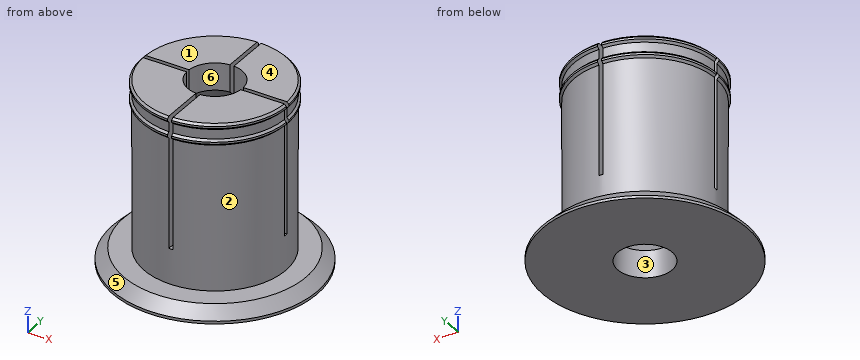
```python
from build123d import *

# Parameters (mm, degrees)
AXLE_BASE_SKETCH_R        = 26
AXLE_DEPTH                = 61.5
GUARD_BASE_R              = 37.5
GUARD_DEPTH               = 5
INNER_AXLE_HOLE_BASE_R    = 10
INNER_AXLE_HOLE_DEPTH     = 67.5
BEND_START                = -48.5
BEND_ROOM_BASE_W          = 1.5
BEND_ROOM_BASE_H          = 75
BEND_ROOM_1_DEPTH         = 48.5
BEND_ROOM_2_COUNT         = 2
BEND_ROOM_2_ANGLE         = 90
EASY_REMOVAL_CHAMFER_SIZE = 4


with BuildPart() as part:
    # Axle base sketch → Axle (new body)
    with BuildSketch(Plane.XY):
        Circle(AXLE_BASE_SKETCH_R)
    extrude(amount=AXLE_DEPTH)

    # Guard base → Guard (add)
    with BuildSketch(Plane(origin=(0, 0, 0), x_dir=(-1, 0, 0), z_dir=(0, 0, -1))):
        Circle(GUARD_BASE_R)
    extrude(amount=GUARD_DEPTH)

    # Inner axle hole base → Inner axle hole (cut, through all)
    with BuildSketch(Plane.XY.offset(61.5)):
        Circle(INNER_AXLE_HOLE_BASE_R)
    extrude(amount=-INNER_AXLE_HOLE_DEPTH, mode=Mode.SUBTRACT)

    # Mate ring base → Mate rings (revolve)
    with BuildSketch(Plane(origin=(0, 0, 0), x_dir=(1, 0, 0), z_dir=(0, 1, 0))):
        Polygon((26, -61.5), (26.75, -60.75), (26.75, -60), (26, -59.25), align=None)
        Polygon((26, -55.75), (26.75, -55), (26.75, -54.25), (26, -53.5), align=None)
    revolve(axis=Axis((0, 0, 0), (0, 0, -1)))

    # Inner mass remove base → Inner mass remove (revolve, cut)
    with BuildSketch(Plane(origin=(0, 0, 0), x_dir=(0, 0, -1), z_dir=(1, 0, 0))):
        Polygon((-61.5, 0), (-43.5, -18), (-13, -18), (5, 0), align=None)
    revolve(axis=Axis((0, 0, 0), (0, 0, -1)), mode=Mode.SUBTRACT)

    # Bend room base → Bend room 1 (cut)
    with BuildSketch(Plane.XY.offset(61.5).offset(BEND_START)):
        Rectangle(BEND_ROOM_BASE_W, BEND_ROOM_BASE_H)
    bend_room_1 = extrude(amount=BEND_ROOM_1_DEPTH, mode=Mode.SUBTRACT)

    # Bend room 2: Bend room 1 ×2 about axis
    bend_room_2_axis = Axis((0, 0, 0), (0, 0, -1))
    for i in range(1, BEND_ROOM_2_COUNT):
        add(bend_room_1.rotate(bend_room_2_axis, i * BEND_ROOM_2_ANGLE / (BEND_ROOM_2_COUNT - 1)), mode=Mode.SUBTRACT)

    # Easy removal chamfer
    easy_removal_chamfer_edges = [part.edges().sort_by_distance(p)[0] for p in [
        (37.5, 0, 0),
    ]]
    chamfer(easy_removal_chamfer_edges, length=EASY_REMOVAL_CHAMFER_SIZE)


solid = part.part
```
For this review, take the finished solid that the model builds, in its own axes (mm). Face numbers are marked on the shaded views. A direction names the side the tool comes from. Round coordinates to 2 decimals unless told otherwise and drop trailing zeros. Write each loop counter-clockwise with the first axis right and the second up, starting at its lowest first coordinate (ties: lowest second). Pieces come first, ordered by that corner, then holes.
1) Insertion check: pin 1 Ø18.5 at (x, z) = (20.5, 36.5) entering from +Y; pin 2 Ø1.2 at (x, y) = (20.5, 0) entering from +Z; pin 3 Ø4 at (x, z) = (-1.5, 30) entering from +Y; pin 4 Ø1.6 at (x, y) = (0, 21) entering from +Z. Each pin has a flat end and moves straight along its axis. Give the tip position at first contact, or say it passes through.
Answer below:
pin 1: stops at y = 23.44
pin 2: stops at z = 13
pin 3: stops at y = 25.99
pin 4: stops at z = 61.5
2) Machinability: for the marked faces 1 and 2, which of the approach directions +Z, -Z, +X, -X, +Y, -Y give a long, thin tool a straight path to every point of the face, cutting with its end or side? Answer none if there is none.
Answer below:
face 1: +Z, +X, -X, +Y, -Y
face 2: none
3) For line 1 along X through (y, z) = (0, 3); line 2 along Z through (x, y) = (-6.5, -25.5), list the stretches that pass through material, from the lowest coordinate up.
Answer below:
line 1: x = -26 to -10, 10 to 26
line 2: z = -5 to 0, 53.82 to 55.43, 59.57 to 61.18
4) Take a section at B-B on z = 49.5. Give the boundary of the cut face in (x, y).
Answer below:
outline: (-25.99, -0.75) arc R26 ccw to (-0.75, -25.99) - (-0.75, -11.98) arc R12 cw to (-11.98, -0.75) - close; (-25.99, 0.75) - (-11.98, 0.75) arc R12 cw to (-0.75, 11.98) - (-0.75, 25.99) arc R26 ccw to start; (0.75, -25.99) arc R26 ccw to (25.99, -0.75) - (11.98, -0.75) arc R12 cw to (0.75, -11.98) - close; (0.75, 11.98) arc R12 cw to (11.98, 0.75) - (25.99, 0.75) arc R26 ccw to (0.75, 25.99) - close
5) Take a section at A-A on z = 19.5. Give the boundary of the cut face in (x, y), then the cut area to 3 significant figures.
Answer below:
outline: (-25.99, -0.75) arc R26 ccw to (-0.75, -25.99) - (-0.75, -17.98) arc R18 cw to (-17.98, -0.75) - close; (-25.99, 0.75) - (-17.98, 0.75) arc R18 cw to (-0.75, 17.98) - (-0.75, 25.99) arc R26 ccw to start; (0.75, -25.99) arc R26 ccw to (25.99, -0.75) - (17.98, -0.75) arc R18 cw to (0.75, -17.98) - close; (0.75, 17.98) arc R18 cw to (17.98, 0.75) - (25.99, 0.75) arc R26 ccw to (0.75, 25.99) - close
area: 1,060 mm2
6) Mouldability with a two-part tool opening along X and no side actions: class the marked faces 3, 4, 5 and 6 as +X half, -X half, draft (parallel to the pull), parting line (faces both ways), or undercut.
Answer below:
face 3: undercut
face 4: draft
face 5: parting line
face 6: undercut
